```python
from build123d import *

# Parameters (mm, degrees)
SKETCH_1_W          = 35
SKETCH_1_H          = 8
EXTRUDE_2_DEPTH     = 8
SKETCH_3_R          = 1.5
CUT_EXTRUDE_1_DEPTH = 8
SKETCH_4_R          = 1.5
CUT_EXTRUDE_2_DEPTH = 8


with BuildPart() as part:
    # 草图1 → 凸台-拉伸2 (new body)
    with BuildSketch(Plane.XY):
        Rectangle(SKETCH_1_W, SKETCH_1_H)
    extrude(amount=EXTRUDE_2_DEPTH)

    # 草图3 → 切除-拉伸1 (cut)
    with BuildSketch(Plane(origin=(0, 0, 0), x_dir=(-1, 0, 0), z_dir=(0, 0, -1))):
        with Locations((-15, 0)):
            Circle(SKETCH_3_R)
        with Locations(Location((15, 0, 0), (0, 0, 180))):
            Circle(SKETCH_3_R)
    extrude(amount=-CUT_EXTRUDE_1_DEPTH, mode=Mode.SUBTRACT)

    # 草图4 → 切除-拉伸2 (cut)
    with BuildSketch(Plane(origin=(0, 4, 0), x_dir=(1, 0, 0), z_dir=(0, 1, 0))):
        with Locations(Location((0, -4, 0), (0, 0, 270))):
            Circle(SKETCH_4_R)
    extrude(amount=-CUT_EXTRUDE_2_DEPTH, mode=Mode.SUBTRACT)


solid = part.part
```
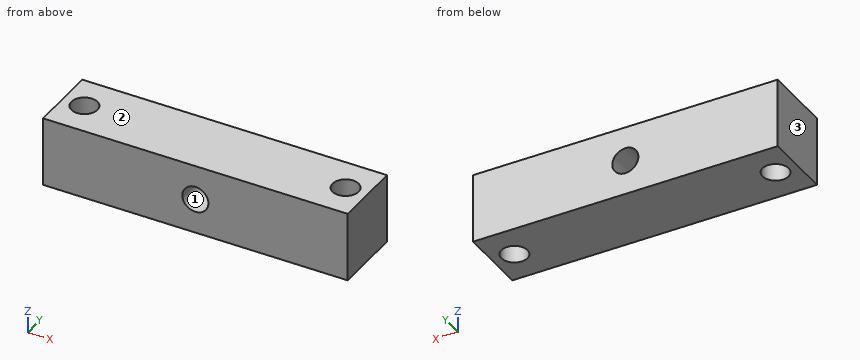
Geometry check sheet. Reference: the model listing, model coordinates, mm. Face numbers are marked on the shaded views. Coordinates: 2 decimals unless noted, no trailing zeros. Loops run counter-clockwise (first coordinate to the right, second up) from the corner with the lowest first, then second, coordinate; pieces in that order, holes last.
Item 1: Sectioned sample at D-D, the plane z = 7. Record the boundary of the cut face in (x, y).
Item 2: Sectioned sample at C-C, the plane x = 0. Record the boundary of the cut face in (y, z), then the cut area to 3 significant figures.
Item 3: Sectioned sample at B-B, the plane y = 0. Record the boundary of the cut face in (x, z).
Item 4: Release check for a two-part mould opening along X. For the marked faces 1, 2 and 3 record: released by +X, released by -X, zero draft, split by the parting line, or undercut.
Item 5: Thickness scan on line 1 (Y direction, x = 15, z = 4.5); line 2 (X direction, y = -1, z = 2); line 3 (Y direction, x = 14, z = 6.75). Record the ranges inside material, lowest first.
Item 6: Sectioned sample at A-A, the plane z = 4. Record the boundary of the cut face in (x, y).
Item 7: Go/stop test with a flat-tipped pin: pin 1 Ø1.8 at (x, y) = (-15, 0) entering from +Z. Record where the tip stops, or that it passes through.
Check result:
1. outline: (-17.5, -4) - (17.5, -4) - (17.5, 4) - (-17.5, 4) - close; hole circle Ø3 at (-15, 0); hole circle Ø3 at (15, 0)
2. outline: (-4, 0) - (4, 0) - (4, 2.5) - (-4, 2.5) - close; (-4, 5.5) - (4, 5.5) - (4, 8) - (-4, 8) - close
2. area: 40.0 mm2
3. outline: (-17.5, 0) - (-16.5, 0) - (-16.5, 8) - (-17.5, 8) - close; (-13.5, 0) - (13.5, 0) - (13.5, 8) - (-13.5, 8) - close; (16.5, 0) - (17.5, 0) - (17.5, 8) - (16.5, 8) - close; hole circle Ø3 at (0, 4)
4. face 1: undercut
4. face 2: zero draft
4. face 3: released by -X
5. line 1: y = -4 to -1.5, 1.5 to 4
5. line 2: x = -17.5 to -16.12, -13.88 to 13.88, 16.12 to 17.5
5. line 3: y = -4 to -1.12, 1.12 to 4
6. outline: (-17.5, -4) - (-1.5, -4) - (-1.5, 4) - (-17.5, 4) - close; (1.5, -4) - (17.5, -4) - (17.5, 4) - (1.5, 4) - close; hole circle Ø3 at (-15, 0); hole circle Ø3 at (15, 0)
7. pin 1: passes through
